The listing builds one solid part. Answer for the finished solid, in the listing's coordinates (mm). A direction names the side the tool comes from. Coordinates: 2 decimals unless noted, no trailing zeros. Loops run counter-clockwise (first coordinate to the right, second up) from the corner with the lowest first, then second, coordinate; pieces in that order, holes last. Notation, with made-up numbers: (20.5, 52) -> (66.5, 52) arc R31 cw to (66.5, 78) -> close; hole circle Ø1 at (51.5, -5.75). An arc over 180 degrees is marked (long way). Answer in a Markdown table with one row per item.
```python
from build123d import *

# Parameters (mm, degrees)
PAD_DEPTH       = 6
SKETCH001_W     = 5.4
SKETCH001_H     = 2.5
SKETCH001_W_2   = 2.7
POCKET_DEPTH    = 224.842404
SKETCH002_R     = 1.7
POCKET001_DEPTH = 224.842404
FILLET_R        = 5


with BuildPart() as part:
    # Sketch → Pad (new body)
    with BuildSketch(Plane.YZ):
        Polygon((-43, 25), (-28, 25), (-28, 0), (28, 0), (28, 25), (43, 25), (43, 15), (49, 15), (49, -7.3), (43, -7.3), (43, -17.3), (33, -17.3), (33, -23.3), (11, -23.3), (11, -17.3), (-11, -17.3), (-11, -23.3), (-33, -23.3), (-33, -17.3), (-43, -17.3), (-43, -7.3), (-49, -7.3), (-49, 15), (-43, 15), align=None)
    extrude(amount=PAD_DEPTH)

    # Sketch001 (on Face25 of Pad) → Pocket (cut, through all)
    with BuildSketch(Plane(origin=(0, 0, 0), x_dir=(0, 1, 0), z_dir=(-1, 0, 0))):
        with Locations((38, 13.05)):
            Rectangle(SKETCH001_W, SKETCH001_H)
        with Locations((1.35, 13.05)):
            Rectangle(SKETCH001_W_2, SKETCH001_H)
    pocket = extrude(amount=-POCKET_DEPTH, mode=Mode.SUBTRACT)

    # Mirrored: Pocket across Sketch001 V_Axis
    add(pocket.mirror(Plane(origin=(0, 0, 0), x_dir=(-1, 0, 0), z_dir=(0, 1, 0))), mode=Mode.SUBTRACT)

    # Sketch002 (on Face4 of Mirrored) → Pocket001 (cut, through all)
    with BuildSketch(Plane(origin=(0, 0, 0), x_dir=(0, 1, 0), z_dir=(-1, 0, 0))):
        with Locations((46, -10)):
            Circle(SKETCH002_R)
        with Locations((46, 2.3)):
            Circle(SKETCH002_R)
    pocket001 = extrude(amount=-POCKET001_DEPTH, mode=Mode.SUBTRACT)

    # Mirrored001: Pocket001 across Sketch002 V_Axis
    add(pocket001.mirror(Plane(origin=(0, 0, 0), x_dir=(-1, 0, 0), z_dir=(0, 1, 0))), mode=Mode.SUBTRACT)

    # Fillet
    fillet_edges = [part.edges().sort_by_distance(p)[0] for p in [
        (3, -28, 0),
        (3, -28, 25),
        (3, 28, 25),
        (3, 28, 0),
    ]]
    fillet(fillet_edges, radius=FILLET_R)


solid = part.part
```
Item 1: A tool of negligible diameter and unlimited length cuts with its end or side. For faces 1 (the face through (3, -27, 2)), 2 (the face through (3, -33, -20)), 3 (the face through (3, -2.7, -13)), from which of +Z, -Z, +X, -X, +Y, -Y can it reach the whole face along a straight path? Write none if from no direction.
Findings below:
| item | result |
|---|---|
| face 1 | +Z, +X, -X |
| face 2 | -Z, +X, -X, -Y |
| face 3 | +X, -X |
Item 2: A cutting plane is placed at D-D, the plane x = 3.8. Count the separate pieces of the cut face and the enclosed holes in it, plus the area to 3 significant figures.
Findings below:
| item | result |
|---|---|
| separate pieces | 1 |
| enclosed holes | 7 |
| area | 2,690 mm2 |
Item 3: A cutting plane is placed at C-C, the plane z = 13.5. Determine the outline of the cut face in (x, y), plus the area to 3 significant figures.
Findings below:
| item | result |
|---|---|
| outline | (0, -49) -> (6, -49) -> (6, -28) -> (0, -28) -> close; (0, 28) -> (6, 28) -> (6, 49) -> (0, 49) -> close |
| area | 252 mm2 |
Item 4: Find the intervals of material crossed by probe 1 along Z at (x, y) = (3.35, -46); probe 2 along Y at (x, z) = (1.45, -2.3); probe 3 along Y at (x, z) = (3.35, 10), in increasing order.
Findings below:
| item | result |
|---|---|
| probe 1 | z = -7.3 to -4, -0.6 to 8.3, 11.7 to 15 |
| probe 2 | y = -49 to -47.7, -44.3 to 44.3, 47.7 to 49 |
| probe 3 | y = -49 to -47.7, -44.3 to -28, 28 to 44.3, 47.7 to 49 |
Item 5: Flat-ended cylindrical pins translate along their axes: pin 1 Ø1.8 at (x, z) = (3, 22) entering from +Y; pin 2 Ø2 at (x, y) = (4.5, -20) entering from +Z; pin 3 Ø3 at (x, y) = (2.5, 47.5) entering from -Z. Find the tip coordinate at first contact, or state that the pin passes through.
Findings below:
| item | result |
|---|---|
| pin 1 | stops at y = 43 |
| pin 2 | stops at z = 0 |
| pin 3 | stops at z = -7.3 |
Item 6: Determine the mould class of faces 4 (the face through (3, 0, 0)), 5 (the face through (3, -35.3, -13)), 6 (the face through (3, -49, 4)), 7 (the face through (3, 49, 4)) for opening direction Y: +Y half, -Y half, draft (parallel to the pull), parting line (faces both ways), or undercut.
Findings below:
| item | result |
|---|---|
| face 4 | undercut |
| face 5 | undercut |
| face 6 | -Y half |
| face 7 | +Y half |
Item 7: A cutting plane is placed at A-A, the plane y = -46. Determine the outline of the cut face in (x, z).
Findings below:
| item | result |
|---|---|
| outline | (0, -7.3) -> (6, -7.3) -> (6, -4) -> (0, -4) -> close; (0, -0.6) -> (6, -0.6) -> (6, 8.3) -> (0, 8.3) -> close; (0, 11.7) -> (6, 11.7) -> (6, 15) -> (0, 15) -> close |
Item 8: A cutting plane is placed at B-B, the plane z = -2.3. Determine the outline of the cut face in (x, y).
Findings below:
| item | result |
|---|---|
| outline | (0, -49) -> (6, -49) -> (6, -47.7) -> (0, -47.7) -> close; (0, -44.3) -> (6, -44.3) -> (6, 44.3) -> (0, 44.3) -> close; (0, 47.7) -> (6, 47.7) -> (6, 49) -> (0, 49) -> close |
